from build123d import *

# Parameters (mm, degrees)
SKETCH016_W     = 22
SKETCH016_H     = 28.9
SKETCH016_R     = 1.25
PAD010_DEPTH    = 7
POCKET005_DEPTH = 4.2
SKETCH020_R     = 2.8
POCKET006_DEPTH = 2.8
SKETCH021_R     = 2.8
PAD011_DEPTH    = 30
SKETCH022_R     = 1.25
POCKET007_DEPTH = 5.3
SKETCH026_W     = 22
SKETCH026_H     = 3
PAD015_DEPTH    = 10


with BuildPart() as part:
    # Sketch016 (on Face1 of ReferencePad007) → Pad010 (new body)
    with BuildSketch(Plane.XY.offset(3.5)):
        with Locations((0, 132.225)):
            Rectangle(SKETCH016_W, SKETCH016_H)
        with Locations((-7.5, 137.225)):
            Circle(SKETCH016_R, mode=Mode.SUBTRACT)
        with Locations((-7.5, 127.225)):
            Circle(SKETCH016_R, mode=Mode.SUBTRACT)
        with Locations((7.5, 137.225)):
            Circle(SKETCH016_R, mode=Mode.SUBTRACT)
        with Locations((7.5, 127.225)):
            Circle(SKETCH016_R, mode=Mode.SUBTRACT)
    extrude(amount=PAD010_DEPTH)

    # Sketch019 (on Face10 of Pad010) → Pocket005 (cut)
    with BuildSketch(Plane.XY.offset(10.5)):
        Polygon((-8.411624, 133.725), (-11, 136.313376), (-11, 146.675), (11, 146.675), (11, 136.313376), (8.411624, 133.725), align=None)
    extrude(amount=-POCKET005_DEPTH, mode=Mode.SUBTRACT)

    # Sketch020 (on Face5 of Pocket005) → Pocket006 (cut)
    with BuildSketch(Plane.XY.offset(10.5)):
        with Locations((-7.5, 127.225)):
            Circle(SKETCH020_R)
        with Locations((7.5, 127.225)):
            Circle(SKETCH020_R)
    extrude(amount=-POCKET006_DEPTH, mode=Mode.SUBTRACT)

    # Sketch021 (on Face5 of Pocket006) → Pad011 (join)
    with BuildSketch(Plane.XY.offset(10.5)):
        Polygon((-4.5, 123.725), (11, 123.725), (11, 133.725), (1.5, 133.725), (1.5, 125.725), (-4.5, 125.725), align=None)
        with Locations((7.5, 127.225)):
            Circle(SKETCH021_R, mode=Mode.SUBTRACT)
    extrude(amount=PAD011_DEPTH)

    # Sketch022 (on Face17 of Pad011) → Pocket007 (cut)
    with BuildSketch(Plane(origin=(1.5, 0, 8), x_dir=(0, -1, 0), z_dir=(-1, 0, 0))):
        with Locations((-130.225, 27.5)):
            Circle(SKETCH022_R)
        with Locations((-130.225, 7.5)):
            Circle(SKETCH022_R)
    extrude(amount=-POCKET007_DEPTH, mode=Mode.SUBTRACT)

    # Sketch026 (on Face5 of Pocket007) → Pad015 (join)
    with BuildSketch(Plane.XY.offset(10.5)):
        with Locations((0, 119.275)):
            Rectangle(SKETCH026_W, SKETCH026_H)
    extrude(amount=PAD015_DEPTH)


solid = part.part
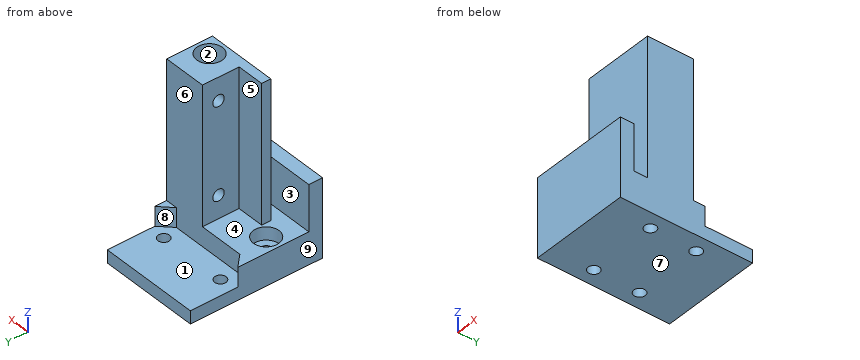
Geometry check sheet. Reference: the model listing, model coordinates, mm. Face numbers are marked on the shaded views. A direction names the side the tool comes from. Give positions to 0.01 mm unless a question says otherwise; leave off trailing zeros. Loops run counter-clockwise (first coordinate to the right, second up) from the corner with the lowest first, then second, coordinate; pieces in that order, holes last. Notation, with made-up numbers: M 45.25,-18.5 L 101.25,-18.5 A26 cw 101.25,-2.5 Z; hole C 40,48.25 d4. An arc over 180 degrees is marked long. Answer as a JSON object with one key per item and string values. Group by question number.
Item 1: Material ranges on L1, parallel to Y at x = -7.5, z = 4.9 (3 decimals); L2, parallel to Y at x = 4, z = 15.5 (3 decimals); L3, parallel to X at y = 128.75, z = 8.5, recorded low to high.
Item 2: Sectioned sample at C-C on x = -0.75. Record the boundary of the cut face in (y, z) (3 decimals).
Item 3: Sectioned sample at B-B on z = 11.5. Record the boundary of the cut face in (x, y) (3 decimals), plus the area to 3 significant figures.
Item 4: Access from +Z, -Z, +X, -X, +Y, -Y to the whole of each face (thin tool, end or side, straight path). Record for the marked faces 1, 2, 3, 4 and 5.
Item 5: Mould release check, pull along X, two halves, no side actions. Record for the marked faces 6, 7, 8 and 9: pulls with the +X half, pulls with the -X half, needs draft (parallel to the pull), parting line crosses it, or undercut.
Item 6: Sectioned sample at A-A on x = -7.5. Record the boundary of the cut face in (y, z) (3 decimals).
Item 7: Gauge pin test, flat ends, axial feed: pin 1 (1 mm diameter, centred on x = -3.5, z = 23.5, fed in from -Y) (3 decimals); pin 2 (0.9 mm diameter, centred on x = -4.5, y = 118.5, fed in from +Z); pin 3 (12 mm diameter, centred on x = -1.5, z = 15, fed in from +Y) (3 decimals). Record the tip position at first contact, or that the pin passes through.
Item 8: Sectioned sample at D-D on z = 27.5. Record the boundary of the cut face in (x, y) (3 decimals), plus the area to 3 significant figures.
Findings below:
{
 "1": {"L1": "117.775 to 125.975, 128.475 to 135.975, 138.475 to 146.675", "L2": "117.775 to 120.775, 123.725 to 128.975, 131.475 to 133.725", "L3": "-11 to -9.85, -5.15 to 5.15, 9.85 to 11"},
 "2": {"outline": "M 117.775,3.5 L 146.675,3.5 L 146.675,6.3 L 133.725,6.3 L 133.725,10.5 L 125.725,10.5 L 125.725,40.5 L 123.725,40.5 L 123.725,10.5 L 120.775,10.5 L 120.775,20.5 L 117.775,20.5 Z"},
 "3": {"outline": "M -11,117.775 L 11,117.775 L 11,120.775 L -11,120.775 Z; M -4.5,123.725 L 11,123.725 L 11,133.725 L 1.5,133.725 L 1.5,125.725 L -4.5,125.725 Z; hole C 7.5,127.225 d5.6", "area": "148 mm2"},
 "4": {"face 1": "+Z, +Y", "face 2": "+Z", "face 3": "+Z, +X, -X", "face 4": "+Z, -X", "face 5": "+Z, -X, +Y"},
 "5": {"face 6": "undercut", "face 7": "needs draft", "face 8": "undercut", "face 9": "pulls with the -X half"},
 "6": {"outline": "M 117.775,3.5 L 125.975,3.5 L 125.975,7.7 L 124.425,7.7 L 124.425,10.5 L 120.775,10.5 L 120.775,20.5 L 117.775,20.5 Z; M 128.475,3.5 L 135.975,3.5 L 135.975,6.3 L 133.725,6.3 L 133.725,10.5 L 130.025,10.5 L 130.025,7.7 L 128.475,7.7 Z; M 138.475,3.5 L 146.675,3.5 L 146.675,6.3 L 138.475,6.3 Z"},
 "7": {"pin 1": "y = 123.725", "pin 2": "z = 20.5", "pin 3": "y = 133.725"},
 "8": {"outline": "M -4.5,123.725 L 11,123.725 L 11,133.725 L 1.5,133.725 L 1.5,125.725 L -4.5,125.725 Z; hole C 7.5,127.225 d5.6", "area": "82.4 mm2"}
}
